from build123d import *

# Parameters (mm, degrees)
PAD_DEPTH    = 6
SKETCH_R     = 12.315
PAD001_DEPTH = 12
SKETCH001_R  = 6.35
POCKET_DEPTH = 18


with BuildPart() as part:
    # Sprocket → Pad (new body)
    with BuildSketch(Plane.XY):
        with BuildLine():
            ThreePointArc((-7.741217, 18.688951), (-5.866931, 17.566734), (-4.442485, 15.910452))
            Line((-4.442485, 15.910452), (-4.167177, 15.46119))
            ThreePointArc((-4.167177, 15.46119), (-3.606611, 14.637889), (-2.969716, 13.872106))
            ThreePointArc((-2.969716, 13.872106), (-1.622244, 12.906521), (0, 12.5654))
            ThreePointArc((0, 12.5654), (1.622244, 12.906521), (2.969716, 13.872106))
            ThreePointArc((2.969716, 13.872106), (3.606611, 14.637889), (4.167177, 15.46119))
            Line((4.167177, 15.46119), (4.442485, 15.910452))
            ThreePointArc((4.442485, 15.910452), (5.866931, 17.566734), (7.741217, 18.688951))
            ThreePointArc((7.741217, 18.688951), (8.27301, 16.570104), (8.109077, 14.391699))
            Line((8.109077, 14.391699), (7.986073, 13.879351))
            ThreePointArc((7.986073, 13.879351), (7.800291, 12.90081), (7.709154, 11.908967))
            ThreePointArc((7.709154, 11.908967), (7.979189, 10.273388), (8.885079, 8.885079))
            ThreePointArc((8.885079, 8.885079), (10.273388, 7.979189), (11.908967, 7.709154))
            Line((11.908967, 7.709154), (13.879351, 7.986073))
            ThreePointArc((13.879351, 7.986073), (14.134744, 8.050827), (14.391699, 8.109077))
            ThreePointArc((14.391699, 8.109077), (16.570104, 8.27301), (18.688951, 7.741217))
            ThreePointArc((18.688951, 7.741217), (17.566734, 5.866931), (15.910452, 4.442485))
            Line((15.910452, 4.442485), (15.46119, 4.167177))
            ThreePointArc((15.46119, 4.167177), (14.637889, 3.606611), (13.872106, 2.969716))
            ThreePointArc((13.872106, 2.969716), (12.906521, 1.622244), (12.5654, 0))
            ThreePointArc((12.5654, 0), (12.906521, -1.622244), (13.872106, -2.969716))
            Line((13.872106, -2.969716), (15.46119, -4.167177))
            ThreePointArc((15.46119, -4.167177), (15.687568, -4.30198), (15.910452, -4.442485))
            ThreePointArc((15.910452, -4.442485), (17.566734, -5.866931), (18.688951, -7.741217))
            ThreePointArc((18.688951, -7.741217), (16.570104, -8.27301), (14.391699, -8.109077))
            Line((14.391699, -8.109077), (13.879351, -7.986073))
            ThreePointArc((13.879351, -7.986073), (12.90081, -7.800291), (11.908967, -7.709154))
            ThreePointArc((11.908967, -7.709154), (10.273388, -7.979189), (8.885079, -8.885079))
            ThreePointArc((8.885079, -8.885079), (7.979189, -10.273388), (7.709154, -11.908967))
            Line((7.709154, -11.908967), (7.986073, -13.879351))
            ThreePointArc((7.986073, -13.879351), (8.050827, -14.134744), (8.109077, -14.391699))
            ThreePointArc((8.109077, -14.391699), (8.27301, -16.570104), (7.741217, -18.688951))
            ThreePointArc((7.741217, -18.688951), (5.866931, -17.566734), (4.442485, -15.910452))
            Line((4.442485, -15.910452), (4.167177, -15.46119))
            ThreePointArc((4.167177, -15.46119), (3.606611, -14.637889), (2.969716, -13.872106))
            ThreePointArc((2.969716, -13.872106), (1.622244, -12.906521), (0, -12.5654))
            ThreePointArc((0, -12.5654), (-1.622244, -12.906521), (-2.969716, -13.872106))
            Line((-2.969716, -13.872106), (-4.167177, -15.46119))
            ThreePointArc((-4.167177, -15.46119), (-4.30198, -15.687568), (-4.442485, -15.910452))
            ThreePointArc((-4.442485, -15.910452), (-5.866931, -17.566734), (-7.741217, -18.688951))
            ThreePointArc((-7.741217, -18.688951), (-8.27301, -16.570104), (-8.109077, -14.391699))
            Line((-8.109077, -14.391699), (-7.986073, -13.879351))
            ThreePointArc((-7.986073, -13.879351), (-7.800291, -12.90081), (-7.709154, -11.908967))
            ThreePointArc((-7.709154, -11.908967), (-7.979189, -10.273388), (-8.885079, -8.885079))
            ThreePointArc((-8.885079, -8.885079), (-10.273388, -7.979189), (-11.908967, -7.709154))
            Line((-11.908967, -7.709154), (-13.879351, -7.986073))
            ThreePointArc((-13.879351, -7.986073), (-14.134744, -8.050827), (-14.391699, -8.109077))
            ThreePointArc((-14.391699, -8.109077), (-16.570104, -8.27301), (-18.688951, -7.741217))
            ThreePointArc((-18.688951, -7.741217), (-17.566734, -5.866931), (-15.910452, -4.442485))
            Line((-15.910452, -4.442485), (-15.46119, -4.167177))
            ThreePointArc((-15.46119, -4.167177), (-14.637889, -3.606611), (-13.872106, -2.969716))
            ThreePointArc((-13.872106, -2.969716), (-12.906521, -1.622244), (-12.5654, 0))
            ThreePointArc((-12.5654, 0), (-12.906521, 1.622244), (-13.872106, 2.969716))
            Line((-13.872106, 2.969716), (-15.46119, 4.167177))
            ThreePointArc((-15.46119, 4.167177), (-15.687568, 4.30198), (-15.910452, 4.442485))
            ThreePointArc((-15.910452, 4.442485), (-17.566734, 5.866931), (-18.688951, 7.741217))
            ThreePointArc((-18.688951, 7.741217), (-16.570104, 8.27301), (-14.391699, 8.109077))
            Line((-14.391699, 8.109077), (-13.879351, 7.986073))
            ThreePointArc((-13.879351, 7.986073), (-12.90081, 7.800291), (-11.908967, 7.709154))
            ThreePointArc((-11.908967, 7.709154), (-10.273388, 7.979189), (-8.885079, 8.885079))
            ThreePointArc((-8.885079, 8.885079), (-7.979189, 10.273388), (-7.709154, 11.908967))
            Line((-7.709154, 11.908967), (-7.986073, 13.879351))
            ThreePointArc((-7.986073, 13.879351), (-8.050827, 14.134744), (-8.109077, 14.391699))
            ThreePointArc((-8.109077, 14.391699), (-8.27301, 16.570104), (-7.741217, 18.688951))
        make_face()
    extrude(amount=PAD_DEPTH)

    # Sketch (on Face50 of Pad) → Pad001 (join)
    with BuildSketch(Plane.XY.offset(6)):
        Circle(SKETCH_R)
    extrude(amount=PAD001_DEPTH)

    # Sketch001 (on Face60 of Pad001) → Pocket (cut)
    with BuildSketch(Plane.XY.offset(18)):
        Circle(SKETCH001_R)
    extrude(amount=-POCKET_DEPTH, mode=Mode.SUBTRACT)


solid = part.part
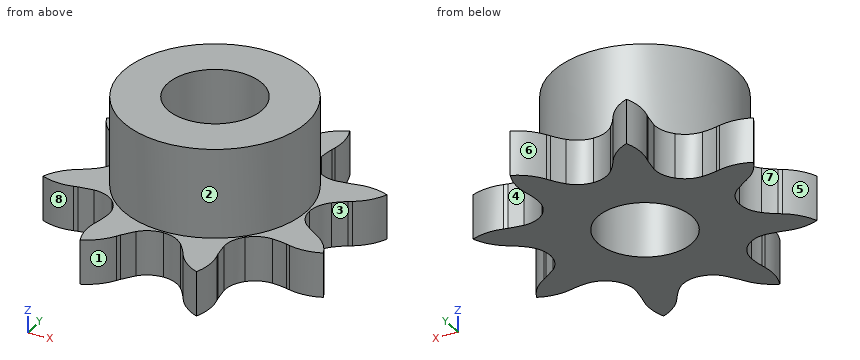
Source: CAD feature listing. Evaluate the final solid. Frame: model axes, mm. Face numbers are marked on the shaded views. A direction names the side the tool comes from. Round coordinates to 2 decimals unless told otherwise and drop trailing zeros. Loops run counter-clockwise (first coordinate to the right, second up) from the corner with the lowest first, then second, coordinate; pieces in that order, holes last.
Q1. Access query for the marked faces 1, 2, 3, 4 and 5. Directions: +Z, -Z, +X, -X, +Y, -Y. A direction counts if a zero-diameter tool reaches every point of the face in a straight line with its end or side. Return the directions, or none.
Q2. Section D-D, the plane x = -10.5. Return loops of the section in (y, z) (3 decimals).
Q3. Section C-C, the plane x = 10. Return loops of the section in (y, z).
Q4. Ray query, line 1 (Y direction, x = 0, z = 14) (3 decimals); line 2 (Z direction, x = -11.5, y = -7); line 3 (Y direction, x = 16, z = 1.75). Return the intervals inside material, ascending.
Q5. Mould query, pull axis Y, two halves, no side actions, for the marked faces 6, 7 and 8. Classes: pulls with the +Y half, pulls with the -Y half, needs draft (parallel to the pull), parting line crosses it, or undercut.
Q6. Section B-B, the plane z = 14.5. Return loops of the section in (x, y) (3 decimals), plus the area to 3 significant figures.
Q7. Section A-A, the plane x = 16.5. Return loops of the section in (y, z).
Q8. First-contact query: P1, Ø2, axis at x = 11, y = 11, coming from the +Z side; P2, Ø5, axis at x = -7.5, y = 3, coming from the -Z side; P3, Ø1.5, axis at x = -3, z = 2.5, coming from the +Y side; P4, Ø6, axis at y = -9, z = 15.5, coming from the -X side. Flat tips, straight axial feed; report the tip coordinate or a pass-through.
Solutions:
1. face 1: +Z, -Z, -Y
1. face 2: +Z
1. face 3: +Z, -Z, +X
1. face 4: +Z, -Z, +Y
1. face 5: +Z, -Z, -X
2. outline: (-7.899, 0) - (7.899, 0) - (7.899, 6) - (6.435, 6) - (6.435, 18) - (-6.435, 18) - (-6.435, 6) - (-7.899, 6) - close
3. outline: (-8.1, 0) - (8.1, 0) - (8.1, 6) - (7.19, 6) - (7.19, 18) - (-7.19, 18) - (-7.19, 6) - (-8.1, 6) - close
4. line 1: y = -12.315 to -6.35, 6.35 to 12.315
4. line 2: z = 0 to 6
4. line 3: y = -8.3 to -4.5, 4.5 to 8.3
5. face 6: pulls with the +Y half
5. face 7: undercut
5. face 8: pulls with the -Y half
6. outline: circle Ø24.63 at (0, 0); hole circle Ø12.7 at (0, 0)
6. area: 350 mm2
7. outline: (-8.28, 0) - (-4.85, 0) - (-4.85, 6) - (-8.28, 6) - close; (4.85, 0) - (8.28, 0) - (8.28, 6) - (4.85, 6) - close
8. P1: passes through
8. P2: stops at z = 0
8. P3: stops at y = 14.83
8. P4: stops at x = -10.75
